Solid Edge part; units mm, degrees
sketch "Sketch1" plane through (0, 0, 0) normal (0, 0, 1) x (1, 0, 0)
  circle A0 centre (0, 0) radius 10
  circle A1 centre (-12.9904, -7.5) radius 1.5
  circle A2 centre (0, 15) radius 1.5
  circle A3 centre (12.9904, -7.5) radius 1.5
  circle A4 centre (0, 0) radius 80
extrude "Protrusion1" add sketch "Sketch1" along normal blind 5
sketch "Sketch2" plane through (0, 0, 5) normal (0, 0, 1) x (1, 0, 0)
  circle A0 centre (0, 15) radius 3
  circle A1 centre (-12.9904, -7.5) radius 3
  circle A2 centre (12.9904, -7.5) radius 3
extrude "ExtrudedCutout_1" cut sketch "Sketch2" against normal blind 2
extrude "ExtrudedCutout_2" [suppressed]
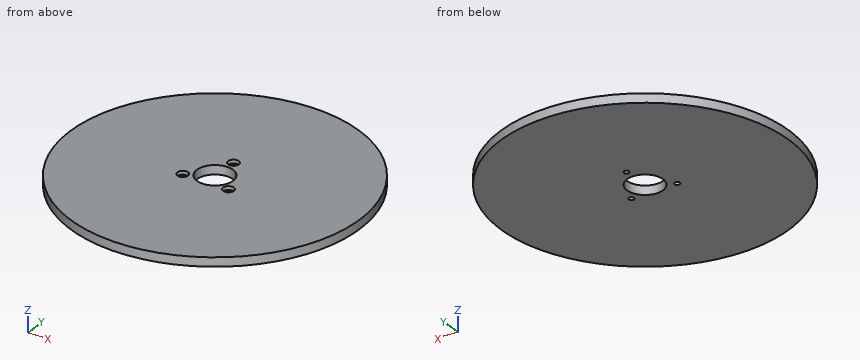
Input: part model. Units: mm. Frame: model coordinates. Coordinates: 2 decimals unless noted, no trailing zeros. Loops run counter-clockwise (first coordinate to the right, second up) from the corner with the lowest first, then second, coordinate; pieces in that order, holes last. Notation, with made-up numbers: M 16.5,63 L 42.5,63 A17 ccw 42.5,73 Z; hole C 20,19.5 d1. An arc over 180 degrees is marked long. Answer in a Markdown table with one row per item.
1. Section B-B, the plane x = -8. Output: boundary loops of the cut face in (y, z), then the cut area to 3 significant figures.
Response:
| item | result |
|---|---|
| outline | M -79.6,0 L -6,0 L -6,5 L -79.6,5 Z; M 6,0 L 79.6,0 L 79.6,5 L 6,5 Z |
| area | 736 mm2 |
2. Section D-D, the plane x = 25. Output: boundary loops of the cut face in (y, z), then the cut area to 3 significant figures.
Response:
| item | result |
|---|---|
| outline | M -75.99,0 L 75.99,0 L 75.99,5 L -75.99,5 Z |
| area | 760 mm2 |
3. First-contact query: pin 1 (5 mm diameter, centred on x = -13, y = -7.5, fed in from +Z); pin 2 (5.5 mm diameter, centred on x = 12.99, y = -7.5, fed in from -Z); pin 3 (3 mm diameter, centred on x = 44.5, z = 1.5, fed in from +Y); pin 4 (3 mm diameter, centred on y = 2.5, z = 1.5, fed in from -X). Flat tips, straight axial feed; report the tip coordinate or a pass-through.
Response:
| item | result |
|---|---|
| pin 1 | stops at z = 3 |
| pin 2 | stops at z = 0 |
| pin 3 | stops at y = 67.46 |
| pin 4 | stops at x = -79.99 |
4. Material intervals for line 1 (X direction, y = -7.5, z = 2.4); line 2 (Y direction, x = 13.5, z = 1); line 3 (X direction, y = 2, z = 1.4) (3 decimals), sorted ascending.
Response:
| item | result |
|---|---|
| line 1 | x = -79.65 to -14.49, -11.49 to -6.61, 6.61 to 11.49, 14.49 to 79.65 |
| line 2 | y = -78.85 to -8.91, -6.09 to 78.85 |
| line 3 | x = -79.975 to -9.798, 9.798 to 79.975 |
5. Section C-C, the plane z = 3.8. Output: boundary loops of the cut face in (x, y), then the cut area to 3 significant figures.
Response:
| item | result |
|---|---|
| outline | C 0,0 d160; hole C -12.99,-7.5 d6; hole C 0,0 d20; hole C 0,15 d6; hole C 12.99,-7.5 d6 |
| area | 19,700 mm2 |
6. Section A-A, the plane y = 0. Output: boundary loops of the cut face in (x, z), then the cut area to 3 significant figures.
Response:
| item | result |
|---|---|
| outline | M -80,0 L -10,0 L -10,5 L -80,5 Z; M 10,0 L 80,0 L 80,5 L 10,5 Z |
| area | 700 mm2 |
